Work out the finished part from the listing and answer in its coordinate system (mm). Face numbers are marked on the shaded views. A direction names the side the tool comes from. Coordinates: 2 decimals unless noted, no trailing zeros. Write each loop counter-clockwise with the first axis right and the second up, starting at its lowest first coordinate (ties: lowest second). Pieces come first, ordered by that corner, then holes. Notation, with made-up numbers: (2, 4) - (51, 4) arc R24 ccw to (51, 30) - close; hole circle Ø6 at (75, -15). An arc over 180 degrees is marked (long way). Use one line per item in the form item = value. Start each with the question number.
Item 1: A cutting plane is placed at A-A (x = 0). Write down the section's boundary in (y, z).
Item 2: Given pin 1 (1.1 mm diameter, centred on y = 43.5, z = 0, fed in from +X); pin 2 (2 mm diameter, centred on x = 0, z = 2.5, fed in from +Y); pin 3 (3 mm diameter, centred on y = 10, z = -3.5, fed in from -X), each flat-ended and moving along its own axis, determine where each tip first touches the part or whether it passes through.
Item 3: A cutting plane is placed at D-D (x = -7.25). Write down the section's boundary in (y, z), then the cut area to 3 significant figures.
Item 4: A cutting plane is placed at B-B (z = 18.5). Write down the section's boundary in (x, y), then the cut area to 3 significant figures.
Item 5: A cutting plane is placed at C-C (y = 28). Write down the section's boundary in (x, z).
Item 6: For the marked faces 1, 2 and 3, determine the directions among +Z, -Z, +X, -X, +Y, -Y from which every point of the face is accessible in a straight line to the end or side of a thin tool.
Item 7: Consider probe 1 along Y at (x, z) = (10.5, 10.5); probe 2 along Z at (x, y) = (11.25, 3); probe 3 along Z at (x, y) = (-5.25, 28). Determine where each line is inside the solid, lowest interval first.
from build123d import *

# Parameters (mm, degrees)
BOSS_EXTRUDE1_DEPTH = 15
SKETCH2_R           = 6.5
BOSS_EXTRUDE2_DEPTH = 22
SKETCH3_R           = 1
BOSS_EXTRUDE3_DEPTH = 3
SKETCH4_W           = 7
SKETCH4_H           = 1
BOSS_EXTRUDE4_DEPTH = 11


with BuildPart() as part:
    # Sketch1 → Boss-Extrude1 (new body)
    with BuildSketch(Plane(origin=(0, 0, 0), x_dir=(1, 0, 0), z_dir=(0, 1, 0))):
        with BuildLine():
            Line((-13, 0), (-13, -21))
            Line((-13, -21), (13, -21))
            Line((13, -21), (13, 0))
            ThreePointArc((13, 0), (0, 13), (-13, 0))
        make_face()
    extrude(amount=BOSS_EXTRUDE1_DEPTH)

    # Sketch2 → Boss-Extrude2 (add)
    with BuildSketch(Plane(origin=(0, 15, 0), x_dir=(1, 0, 0), z_dir=(0, 1, 0))):
        with Locations(Location((0, 0, 0), (0, 0, 270))):
            Circle(SKETCH2_R)
    extrude(amount=BOSS_EXTRUDE2_DEPTH)

    # Sketch3 → Boss-Extrude3 (add)
    with BuildSketch(Plane(origin=(0, 37, 0), x_dir=(1, 0, 0), z_dir=(0, 1, 0))):
        with Locations(Location((0, 0, 0), (0, 0, 270))):
            Circle(SKETCH3_R)
    extrude(amount=BOSS_EXTRUDE3_DEPTH)

    # Sketch4 → Boss-Extrude4 (add)
    with BuildSketch(Plane(origin=(0, 40, 0), x_dir=(1, 0, 0), z_dir=(0, 1, 0))):
        Rectangle(SKETCH4_W, SKETCH4_H)
    extrude(amount=BOSS_EXTRUDE4_DEPTH)


solid = part.part
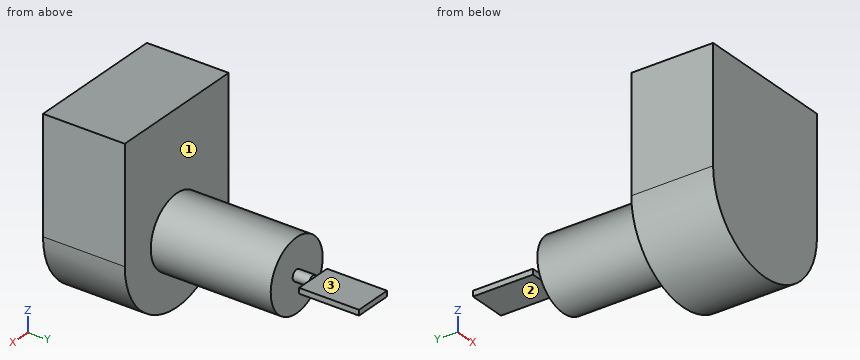
Answer:
q1.outline = (0, -13) - (15, -13) - (15, -6.5) - (37, -6.5) - (37, -1) - (40, -1) - (40, -0.5) - (51, -0.5) - (51, 0.5) - (40, 0.5) - (40, 1) - (37, 1) - (37, 6.5) - (15, 6.5) - (15, 21) - (0, 21) - close
q2.pin_1 = 3.5
q2.pin_2 = 37
q2.pin_3 = -12.85
q3.outline = (0, -10.79) - (15, -10.79) - (15, 21) - (0, 21) - close
q3.area = 477 mm²
q4.outline = (-13, 0) - (13, 0) - (13, 15) - (-13, 15) - close
q4.area = 390 mm²
q5.outline = circle Ø13 at (0, 0)
q6.face_1 = +Y
q6.face_2 = -Z, +X, -X, +Y
q6.face_3 = +Z, +X, -X, +Y
q7.probe_1 = 0 to 15
q7.probe_2 = -6.51 to 21
q7.probe_3 = -3.83 to 3.83
